Study the drawing (mm; zero at the part's minimum x, y, z) and answer. A direction names the side the tool comes from. Round coordinates to 2 decimals unless told otherwise and drop trailing zeros. Write each loop counter-clockwise with the first axis right and the second up, starting at its lowest first coordinate (ties: lowest second). Pieces come first, ordered by that corner, then holes. Notation, with made-up numbers: M 71,59 L 127,59 A14 cw 127,69 Z; hole C -21,5 d11. An arc over 180 degrees is marked long. Write each question's results on one line, items separated by ' | '.
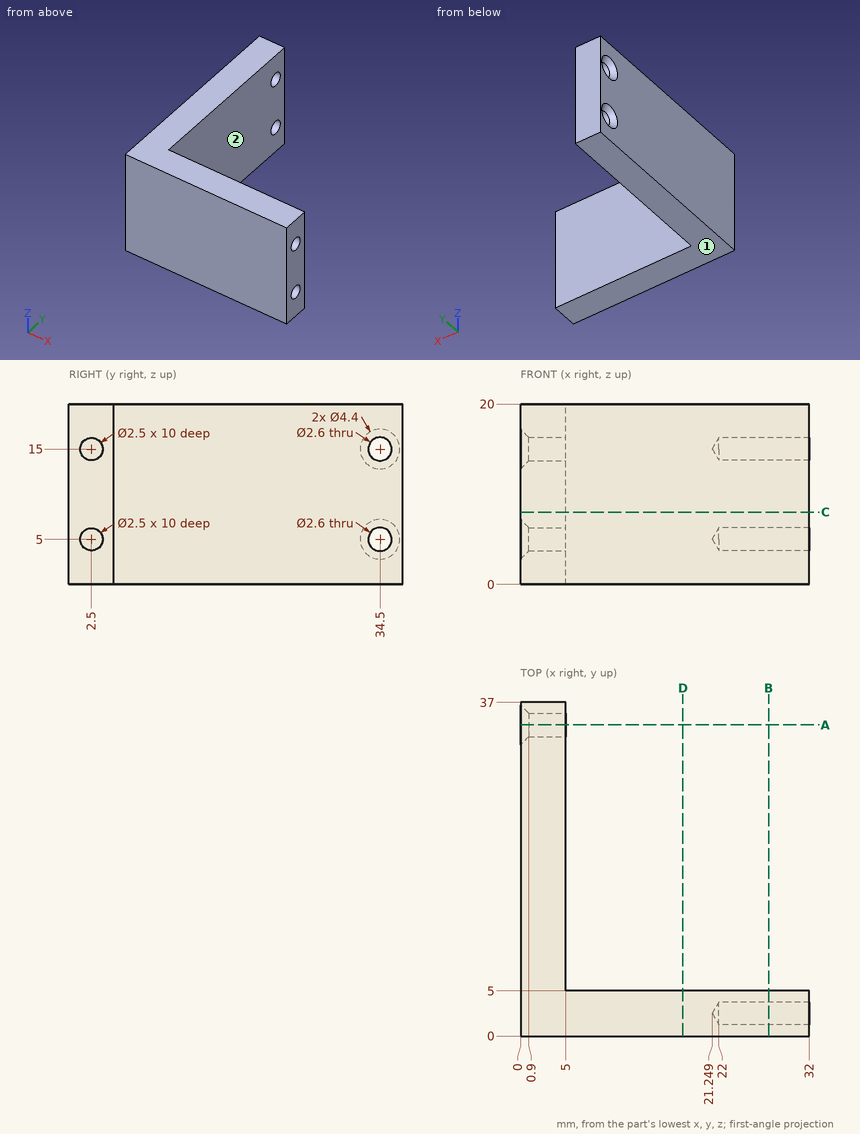
1) Section B-B (x = 27.5) is taken. Determine the outline of the cut face in (y, z), then the cut area to 3 significant figures.
Return value:
outline: M 0,0 L 5,0 L 5,20 L 0,20 Z; hole C 2.5,5 d2.5; hole C 2.5,15 d2.5 | area: 90.2 mm²
2) Section C-C (z = 8) is taken. Determine the outline of the cut face in (x, y).
Return value:
outline: M 0,0 L 32,0 L 32,5 L 5,5 L 5,37 L 0,37 Z
3) Each of these flat-tipped pins is pushed along its axis until it touches: pin 1 (3.5 mm diameter, centred on y = 34.5, z = 5, fed in from -X); pin 2 (1.5 mm diameter, centred on x = 13.5, z = 16, fed in from +Y); pin 3 (12 mm diameter, centred on x = 14, z = 12.5, fed in from -Y); pin 4 (10 mm diameter, centred on y = 31, z = 9, fed in from +X). Where does it stop, or does it pass through?
Return value:
pin 1: x = 0.45 | pin 2: y = 5 | pin 3: y = 0 | pin 4: x = 5
4) Section D-D (x = 18) is taken. Determine the outline of the cut face in (y, z), then the cut area to 3 significant figures.
Return value:
outline: M 0,0 L 5,0 L 5,20 L 0,20 Z | area: 100 mm²
5) A tool of negligible diameter and unlimited length cuts with its end or side. For the marked faces 1 and 2, from which of +Z, -Z, +X, -X, +Y, -Y can it reach the whole face along a straight path? Write none if from no direction.
Return value:
face 1: -Z, +X, -X, +Y, -Y | face 2: +Z, -Z, +X, +Y
6) Section A-A (y = 34.5) is taken. Determine the outline of the cut face in (x, z).
Return value:
outline: M 0,0 L 5,0 L 5,3.7 L 0.9,3.7 L 0,2.8 Z; M 0,7.2 L 0.9,6.3 L 5,6.3 L 5,13.7 L 0.9,13.7 L 0,12.8 Z; M 0,17.2 L 0.9,16.3 L 5,16.3 L 5,20 L 0,20 Z
7) Find the intervals of material crossed by line 1 (Z direction, x = 2.4, y = 34.5); line 2 (Z direction, x = 25.25, y = 2.5); line 3 (Y direction, x = 26.75, z = 15), in increasing order.
Return value:
line 1: 0 to 3.7, 6.3 to 13.7, 16.3 to 20 | line 2: 0 to 3.75, 6.25 to 13.75, 16.25 to 20 | line 3: 0 to 1.25, 3.75 to 5
